Can you work these out from the model? Positions are in its coordinate system, mm. A direction names the side the tool comes from. Round coordinates to 2 decimals unless told otherwise and drop trailing zeros. Loops run counter-clockwise (first coordinate to the right, second up) from the corner with the lowest first, then second, coordinate; pieces in that order, holes last.
(1) I want a section at A-A on x = 20.5. Write out the boundary of the cut face in (y, z), plus the area to 3 significant figures.
(2) I want a section at B-B on y = -28. Write out the boundary of the cut face in (x, z), plus the area to 3 significant figures.
(3) If I drill on line 1 along Z through (x, y) = (33, -72), over which ranges is the centre line in solid material (lowest first)?
(4) Which directions (+Z, -Z, +X, -X, +Y, -Y) give clear straight access to the entire face, cutting with the end or side of a thin tool? Please do faces 1 (the face through (60, -45, 9)), 2 (the face through (30, 0, 22)).
(5) Will these pins go through, and if not, where does the flat tip stop? pin 1 Ø18 at (x, y) = (37.5, -59.5) entering from +Z; pin 2 Ø3 at (y, z) = (-33.5, 8.5) entering from -X; pin 3 Ø12.5 at (x, z) = (37, 23) entering from -Y.
from build123d import *

# Parameters (mm, degrees)
BOX002_W     = 60
BOX002_H     = 40
BOX002_DEPTH = 10
BOX001_W     = 60
BOX001_H     = 10
BOX001_DEPTH = 25
BOX_W        = 60
BOX_H        = 100
BOX_DEPTH    = 10


with BuildPart() as cubo002:
    # Box002 → Box002 (new body)
    with BuildSketch(Plane(origin=(0, -130, 0), x_dir=(1, 0, 0), z_dir=(0, 0, 1))):
        with Locations((30, 20)):
            Rectangle(BOX002_W, BOX002_H)
    extrude(amount=BOX002_DEPTH)


with BuildPart() as cubo001:
    # Box001 → Box001 (new body)
    with BuildSketch(Plane.XY.offset(10)):
        with Locations((30, 5)):
            Rectangle(BOX001_W, BOX001_H)
    extrude(amount=BOX001_DEPTH)


with BuildPart() as fusion001:
    # Box → Box (new body)
    with BuildSketch(Plane(origin=(0, -90, 0), x_dir=(1, 0, 0), z_dir=(0, 0, 1))):
        with Locations((30, 50)):
            Rectangle(BOX_W, BOX_H)
    extrude(amount=BOX_DEPTH)

    # Fusion: union Cubo001
    add(cubo001.part)

    # Fusion001: union Cubo002
    add(cubo002.part)


solid = fusion001.part
Filled sheet:
1. outline: (-130, 0) - (10, 0) - (10, 35) - (0, 35) - (0, 10) - (-130, 10) - close
1. area: 1,650 mm2
2. outline: (0, 0) - (60, 0) - (60, 10) - (0, 10) - close
2. area: 600 mm2
3. line 1: z = 0 to 10
4. face 1: +Z, -Z, +X, +Y, -Y
4. face 2: +Z, +X, -X, -Y
5. pin 1: stops at z = 10
5. pin 2: stops at x = 0
5. pin 3: stops at y = 0
